Source: CAD feature listing. Evaluate the final solid. Frame: model axes, mm. Give positions to 0.01 mm unless a question says otherwise; leave off trailing zeros. Write each loop counter-clockwise with the first axis right and the second up, starting at its lowest first coordinate (ties: lowest second). Pieces come first, ordered by that corner, then holes. Notation, with made-up numbers: M -11.5,-17 L -2.5,-17 A18 ccw -2.5,15 Z; hole C 34,-22 d5. An arc over 180 degrees is marked long. Use CSV: the item, a comma, the result in double quotes. Start each with the question number.
from build123d import *

# Parameters (mm, degrees)
SKETCH3_R           = 2.5
SKETCH3_R_2         = 1.5
BOSS_EXTRUDE1_DEPTH = 3.125
FILLET1_R           = 10
SKETCH4_W           = 12.5
SKETCH4_H           = 4
SKETCH4_W_2         = 9
SKETCH4_H_2         = 21
CUT_EXTRUDE2_DEPTH  = 73.594873269


with BuildPart() as part:
    # Sketch3 → Boss-Extrude1 (new body)
    with BuildSketch(Plane.XY):
        with BuildLine():
            Line((0, 23.314265754), (0, 40.6))
            Line((0, 40.6), (1.75, 40.6))
            Line((1.75, 40.6), (1.75, 60.5))
            Line((1.75, 60.5), (40, 60.5))
            Line((40, 60.5), (40, 55.5))
            Line((40, 55.5), (11.73, 55.5))
            Line((11.73, 55.5), (11.73, 43.67))
            Line((11.73, 43.67), (8.55, 43.67))
            Line((8.55, 43.67), (8.55, 40.49))
            Line((8.55, 40.49), (11.73, 40.49))
            Line((11.73, 40.49), (11.73, 37.16))
            Line((11.73, 37.16), (22, 37.16))
            ThreePointArc((22, 37.16), (25.665, 33.495), (22, 29.83))
            Line((22, 29.83), (11.73, 29.83))
            Line((11.73, 29.83), (11.73, 11.5))
            Line((11.73, 11.5), (40, 11.5))
            Line((40, 11.5), (40, -28.5))
            Line((40, -28.5), (21.91, -28.5))
            Line((21.91, -28.5), (21.91, -39.5))
            Line((21.91, -39.5), (18.73, -39.5))
            Line((18.73, -39.5), (18.73, -51.5))
            Line((18.73, -51.5), (21.91, -51.5))
            Line((21.91, -51.5), (21.91, -60.5))
            Line((21.91, -60.5), (12.73, -60.5))
            Line((12.73, -60.5), (12.73, -57.32))
            Line((12.73, -57.32), (9.55, -57.32))
            Line((9.55, -57.32), (9.55, -60.5))
            Line((9.55, -60.5), (0, -60.5))
            Line((0, -60.5), (0, 23.314265754))
        make_face()
        with Locations((22, 33.495)):
            Circle(SKETCH3_R, mode=Mode.SUBTRACT)
        with Locations((30, -4.33)):
            Circle(SKETCH3_R_2, mode=Mode.SUBTRACT)
    boss_extrude1 = extrude(amount=BOSS_EXTRUDE1_DEPTH)

    # Mirror1: Boss-Extrude1 across plane
    add(boss_extrude1.mirror(Plane(origin=(0, 23.314265754, 3.125), x_dir=(0, 0, 1), z_dir=(1, 0, 0))))

    # Fillet1
    # the kernel refuses this fillet: 10 mm, written as the material it takes off along each edge
    with BuildSketch(Plane(origin=(40, 60.5, -21.650635095), x_dir=(0, -1, 0), z_dir=(0, 0, 1))) as fillet1_piece_1:
        with BuildLine():
            CenterArc((10, -8.660254038), FILLET1_R, 120, 60)
            Line((0, -8.660254038), (-0.2, -8.660254038))
            Line((-0.2, -8.660254038), (-0.2, 0))
            Line((-0.2, 0), (0, 0.2))
            ThreePointArc((0, 0.2), (2.5, 0.2), (4.9, 0.173205081))
            Line((4.9, 0.173205081), (5, 0))
        make_face()
    extrude(amount=46.426270189, mode=Mode.SUBTRACT)
    with BuildSketch(Plane(origin=(40, 11.5, -25), x_dir=(0, -1, 0), z_dir=(0, 0, 1)), Plane(origin=(40, -28.5, -25), x_dir=(-1, 0, 0), z_dir=(0, 0, 1)), Plane(origin=(-40, 11.5, -25), x_dir=(1, 0, 0), z_dir=(0, 0, 1)), Plane(origin=(-40, -28.5, -25), x_dir=(0, 1, 0), z_dir=(0, 0, 1))) as fillet1_piece_2:
        with BuildLine():
            CenterArc((FILLET1_R, -FILLET1_R), FILLET1_R, 90, 90)
            Line((0, -FILLET1_R), (-FILLET1_R * 0.02, -FILLET1_R))
            Line((-FILLET1_R * 0.02, -FILLET1_R), (-FILLET1_R * 0.02, FILLET1_R * 0.02))
            Line((-FILLET1_R * 0.02, FILLET1_R * 0.02), (FILLET1_R, FILLET1_R * 0.02))
            Line((FILLET1_R, FILLET1_R * 0.02), (FILLET1_R, 0))
        make_face()
    extrude(amount=53.125, mode=Mode.SUBTRACT)
    with BuildSketch(Plane(origin=(-40, 60.5, -21.650635095), x_dir=(1, 0, 0), z_dir=(0, 0, 1))) as fillet1_piece_3:
        with BuildLine():
            CenterArc((8.660254038, -10), FILLET1_R, 90, 60)
            Line((0, -5), (-0.173205081, -4.9))
            ThreePointArc((-0.173205081, -4.9), (-0.2, -2.5), (-0.2, 0))
            Line((-0.2, 0), (0, 0.2))
            Line((0, 0.2), (8.660254038, 0.2))
            Line((8.660254038, 0.2), (8.660254038, 0))
        make_face()
    extrude(amount=46.426270189, mode=Mode.SUBTRACT)

    # Sketch4 → Cut-Extrude2 (cut, through all)
    with BuildSketch(Plane.XY.offset(3.125)):
        with Locations((0, 28.5)):
            Rectangle(SKETCH4_W, SKETCH4_H)
        with Locations((-12.61, -45.2)):
            Rectangle(SKETCH4_W_2, SKETCH4_H_2)
        with BuildLine():
            Line((-4, -15.06), (4, -15.06))
            ThreePointArc((4, -15.06), (4.707106781, -15.352893219), (5, -16.06))
            Line((5, -16.06), (5, -17.06))
            ThreePointArc((5, -17.06), (4.707106781, -17.767106781), (4, -18.06))
            Line((4, -18.06), (-4, -18.06))
            ThreePointArc((-4, -18.06), (-4.707106781, -17.767106781), (-5, -17.06))
            Line((-5, -17.06), (-5, -16.06))
            ThreePointArc((-5, -16.06), (-4.707106781, -15.352893219), (-4, -15.06))
        make_face()
    extrude(amount=-CUT_EXTRUDE2_DEPTH, mode=Mode.SUBTRACT)


solid = part.part
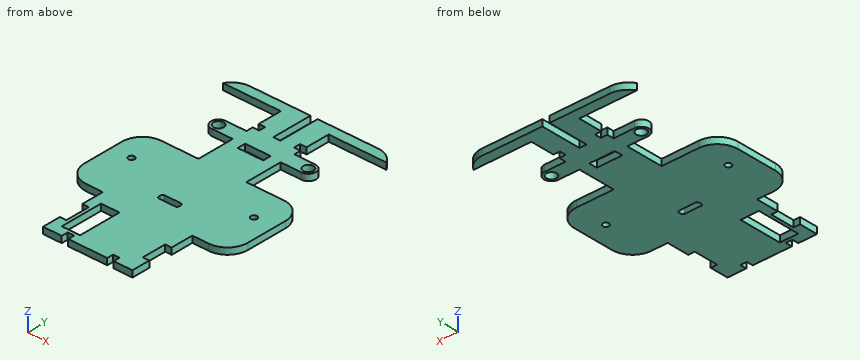
Item 1: Section B-B (x = 15). Return the cut outline in (y, z) (3 decimals).
Item 2: Section D-D (y = -26). Return the cut outline in (x, z) (3 decimals), plus the area to 3 significant figures.
Item 3: Material intervals for probe 1 along Y at (x, z) = (30, 1); probe 2 along Y at (x, z) = (-13, 1.25); probe 3 along Y at (x, z) = (16, 1.9), sorted ascending.
Item 4: Contact query for flat-ended pins moving along their axis: pin 1 Ø2 at (x, y) = (-23.5, 39.5) entering from -Z; pin 2 Ø1.6 at (y, z) = (-59, 2) entering from -X; pin 3 Ø0.9 at (y, z) = (47.5, 1) entering from +X. Output: stop coordinate, or through.
Item 5: Section C-C (z = 1.85). State how many separate pieces and enclosed holes the cut face has, plus the area to 3 significant figures.
Item 6: Section A-A (y = -4.33). Return the cut outline in (x, z) (3 decimals), plus the area to 3 significant figures.
Output values:
1,outline,"M -60.5,0 L 11.5,0 L 11.5,3.125 L -60.5,3.125 Z; M 29.83,0 L 37.16,0 L 37.16,3.125 L 29.83,3.125 Z; M 55.5,0 L 60.5,0 L 60.5,3.125 L 55.5,3.125 Z"
2,outline,"M -36.614,0 L 36.614,0 L 36.614,3.125 L -36.614,3.125 Z"
2,area,"229 mm2"
3,probe 1,"y = -28.5 to -5.83, -2.83 to 11.5, 55.5 to 60.5"
3,probe 2,"y = -60.5 to -55.7, -34.7 to 11.5, 29.83 to 37.16, 55.5 to 60.5"
3,probe 3,"y = -60.5 to 11.5, 29.83 to 37.16, 55.5 to 60.5"
4,pin 1,"passes through"
4,pin 2,"stops at x = -21.91"
4,pin 3,"stops at x = 11.73"
5,separate pieces,"1"
5,enclosed holes,"7"
5,area,"5,610 mm2"
6,outline,"M -40,0 L -31.5,0 L -31.5,3.125 L -40,3.125 Z; M -28.5,0 L 28.5,0 L 28.5,3.125 L -28.5,3.125 Z; M 31.5,0 L 40,0 L 40,3.125 L 31.5,3.125 Z"
6,area,"231 mm2"
